Verification items for the finished model (mm, model axes). Face numbers are marked on the shaded views. A direction names the side the tool comes from. Give positions to 0.01 mm unless a question says otherwise; leave off trailing zeros. Order: outer loops, then holes, each group sorted by start corner. A loop starts at its lowest first (then second) coordinate and runs counter-clockwise, first axis right, second up. Notation, with made-up numbers: (-15.5, 50) - (14.5, 50) arc R12 cw to (14.5, 66) - close; hole circle Ø6 at (15, -14.75). An arc over 180 degrees is marked (long way). Answer as a JSON object with one key per item and string values. Group by question number.
(1) Section check B-B (x = 0). Record the boundary of the cut face in (y, z).
(2) Mould release check, pull along X, two halves, no side actions. Record for the marked faces 3, 4 and 5: +X half, -X half, draft (parallel to the pull), parting line (faces both ways), or undercut.
(3) Access from +Z, -Z, +X, -X, +Y, -Y to the whole of each face (thin tool, end or side, straight path). Record for the marked faces 1 and 2.
(4) Section check D-D (y = 3.25). Record the boundary of the cut face in (x, z), then the cut area to 3 significant figures.
(5) Depth check by flat-ended pin: pin 1 Ø6 at (x, y) = (-3.5, 4) entering from -Z (3 decimals); pin 2 Ø5 at (x, z) = (-0.5, 0.5) entering from +Y; pin 3 Ø6 at (x, y) = (7, 7.5) entering from +Z. Enter the tip coordinate at first touch or a pass-through.
(6) Section check A-A (z = 0). Record the boundary of the cut face in (x, y).
(7) Thickness scan on line 1 (Y direction, x = 4, z = -1.75); line 2 (Z direction, x = -5, y = 8); line 3 (X direction, y = 8.5, z = -5). Record the ranges inside material, lowest first.
(8) Section check C-C (y = 9.75). Record the boundary of the cut face in (x, z), then the cut area to 3 significant figures.
```python
from build123d import *


with BuildPart() as part:
    # Sketch1 → Revolve1 (revolve)
    with BuildSketch(Plane(origin=(0, 0, 0), x_dir=(0, 0, -1), z_dir=(1, 0, 0))):
        with BuildLine():
            Line((0, 0), (11.176, 0))
            Line((11.176, 0), (9.90175141, 9.066749838))
            ThreePointArc((9.90175141, 9.066749838), (9.477305929, 9.848481167), (8.644110962, 10.16))
            Line((8.644110962, 10.16), (6.897941597, 10.16))
            ThreePointArc((6.897941597, 10.16), (6.06474663, 9.848481167), (5.64030115, 9.066749838))
            Line((5.64030115, 9.066749838), (5.08, 5.08))
            Line((5.08, 5.08), (0, 5.08))
            Line((0, 5.08), (0, 0))
        make_face()
    revolve(axis=Axis((0, 0, 0), (0, 1, 0)))


solid = part.part
```
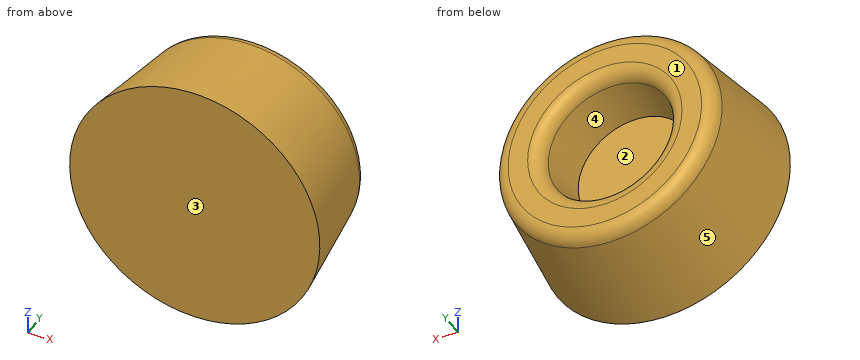
Solutions:
{
 "1": {"outline": "(0, -11.18) - (9.07, -9.9) arc R1.27 ccw to (10.16, -8.64) - (10.16, -6.9) arc R1.27 ccw to (9.07, -5.64) - (5.08, -5.08) - (5.08, 5.08) - (9.07, 5.64) arc R1.27 ccw to (10.16, 6.9) - (10.16, 8.64) arc R1.27 ccw to (9.07, 9.9) - (0, 11.18) - close"},
 "2": {"face 3": "draft", "face 4": "undercut", "face 5": "parting line"},
 "3": {"face 1": "+Z, -Z, +X, -X, +Y", "face 2": "+Y"},
 "4": {"outline": "circle Ø21.44 at (0, 0)", "area": "361 mm2"},
 "5": {"pin 1": "stops at z = -10.825", "pin 2": "stops at y = 5.08", "pin 3": "stops at z = 9.38"},
 "6": {"outline": "(-11.18, 0) - (11.18, 0) - (9.9, 9.07) arc R1.27 ccw to (8.64, 10.16) - (6.9, 10.16) arc R1.27 ccw to (5.64, 9.07) - (5.08, 5.08) - (-5.08, 5.08) - (-5.64, 9.07) arc R1.27 ccw to (-6.9, 10.16) - (-8.64, 10.16) arc R1.27 ccw to (-9.9, 9.07) - close"},
 "7": {"line 1": "y = 0 to 5.08", "line 2": "z = -8.72 to -2.27, 2.27 to 8.72", "line 3": "x = -8.64 to -2.43, 2.43 to 8.64"},
 "8": {"outline": "circle Ø19.16 at (0, 0); hole circle Ø11.93 at (0, 0)", "area": "177 mm2"}
}
